Design review of the part built by this model. Coordinates are the model's own, in mm. Face numbers are marked on the shaded views. A direction names the side the tool comes from. Coordinates: 2 decimals unless noted, no trailing zeros. Write each loop counter-clockwise with the first axis right and the second up, starting at its lowest first coordinate (ties: lowest second). Pieces come first, ordered by that corner, then holes.
Q1. The part is to be moulded in two halves that separate along Z. For the marked faces 3, 4 and 5, say which applies: +Z half, -Z half, draft (parallel to the pull), parting line (faces both ways), or undercut.
Q2. Add section D-D, the plane y = 1.25. Give the boundary of the cut face in (x, z), plus the area to 3 significant figures.
Q3. Add section B-B, the plane y = 14.25. Give the boundary of the cut face in (x, z), plus the area to 3 significant figures.
Q4. Add section A-A, the plane x = 0. Give the boundary of the cut face in (y, z) (3 decimals), plus the area to 3 significant figures.
Q5. Clearance check with flat-ended pins moving along their axes: pin 1 Ø8 at (y, z) = (6, -4.5) entering from -X; pin 2 Ø7.5 at (y, z) = (16.5, 2.5) entering from +X; pin 3 Ø2 at (x, y) = (1.5, 12) entering from +Z. State where each tip first meets the part, or that it passes through.
Q6. To check wall thickness, follow probe 1 along Y at (x, z) = (-0.25, 0); probe 2 along Y at (x, z) = (2, -1.5); probe 3 along X at (y, z) = (3.75, -9). State the ranges of each line that lie inside material, in increasing order.
Q7. Machinability: for the marked faces 1 and 2, which of the approach directions +Z, -Z, +X, -X, +Y, -Y give a long, thin tool a straight path to every point of the face, cutting with its end or side? Answer none if there is none.
Q8. Add section C-C, the plane z = 0. Give the boundary of the cut face in (x, y) (3 decimals), plus the area to 3 significant figures.
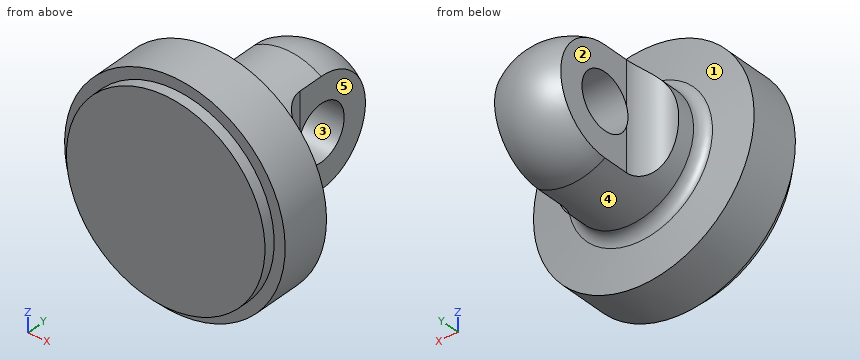
from build123d import *

# Parameters (mm, degrees)
CUT_EXTRUDE1_DEPTH      = 30.071628781
CUT_EXTRUDE1_DEPTH_BACK = 30.071628781
CUT_EXTRUDE2_DEPTH      = 31.926520981
CUT_EXTRUDE2_DEPTH_BACK = 31.926520981
SKETCH4_R               = 3.175


with BuildPart() as part:
    # Sketch1 → Revolve1 (revolve)
    with BuildSketch(Plane.XY, mode=Mode.PRIVATE) as revolve1_sk:
        with BuildLine():
            Line((-12.7, 0), (-12.7, 5.715))
            Line((-12.7, 5.715), (-8.325216792, 6.220171271))
            ThreePointArc((-8.325216792, 6.220171271), (-7.522765602, 6.636837464), (-7.2009, 7.481787854))
            Line((-7.2009, 7.481787854), (-7.2009, 15.6591))
            ThreePointArc((-7.2009, 15.6591), (-5.091805221, 20.750905221), (0, 22.86))
            Line((0, 22.86), (0, 6.35))
            Line((0, 6.35), (0, 0))
            Line((0, 0), (0, -1.27))
            Line((0, -1.27), (-11.43, -1.27))
            Line((-11.43, -1.27), (-11.43, 0))
            Line((-11.43, 0), (-12.7, 0))
        make_face()
    revolve(revolve1_sk.sketch.rotate(Axis((0, 6.35, 0), (0, -1, 0)), 270), axis=Axis((0, 6.35, 0), (0, -1, 0)))

    # Sketch3 → Cut-Extrude1 (cut, two sides: drawn at the far end of the back side and taken through both)
    with BuildSketch(Plane.XY.offset(-CUT_EXTRUDE1_DEPTH_BACK)):
        with BuildLine():
            Line((-3.81, 22.86), (-3.81, 12.7))
            ThreePointArc((-3.81, 12.7), (-6.985, 9.525), (-10.16, 12.7))
            Line((-10.16, 12.7), (-10.16, 22.86))
            Line((-10.16, 22.86), (-3.81, 22.86))
        make_face()
        with BuildLine():
            Line((10.16, 22.86), (10.16, 12.7))
            ThreePointArc((10.16, 12.7), (6.985, 9.525), (3.81, 12.7))
            Line((3.81, 12.7), (3.81, 22.86))
            Line((3.81, 22.86), (10.16, 22.86))
        make_face()
    extrude(amount=CUT_EXTRUDE1_DEPTH + CUT_EXTRUDE1_DEPTH_BACK, mode=Mode.SUBTRACT)

    # Sketch4 → Cut-Extrude2 (cut, two sides: drawn at the far end of the back side and taken through both)
    with BuildSketch(Plane.ZY.offset(3.81).offset(-CUT_EXTRUDE2_DEPTH_BACK)):
        with Locations(Location((0, 15.6591, 0), (0, 0, 248.748756024))):
            Circle(SKETCH4_R)
    extrude(amount=CUT_EXTRUDE2_DEPTH + CUT_EXTRUDE2_DEPTH_BACK, mode=Mode.SUBTRACT)


solid = part.part
Here are the results:
1. face 3: undercut
1. face 4: parting line
1. face 5: draft
2. outline: circle Ø25.4 at (0, 0)
2. area: 507 mm2
3. outline: (-3.81, -6.11) arc R7.2 ccw to (3.81, -6.11) - (3.81, -2.85) - (-3.81, -2.85) - close; (-3.81, 2.85) - (3.81, 2.85) - (3.81, 6.11) arc R7.2 ccw to (-3.81, 6.11) - close
3. area: 61.0 mm2
4. outline: (-1.27, -11.43) - (0, -11.43) - (0, -12.7) - (5.715, -12.7) - (6.22, -8.325) arc R1.27 cw to (7.482, -7.201) - (15.659, -7.201) arc R7.201 ccw to (15.659, 7.201) - (7.482, 7.201) arc R1.27 cw to (6.22, 8.325) - (5.715, 12.7) - (0, 12.7) - (0, 11.43) - (-1.27, 11.43) - close; hole circle Ø6.35 at (15.659, 0)
4. area: 371 mm2
5. pin 1: stops at x = -12.69
5. pin 2: stops at x = 3.81
5. pin 3: stops at z = 7.18
6. probe 1: y = -1.27 to 12.48, 18.83 to 22.86
6. probe 2: y = -1.27 to 12.86, 18.46 to 22.41
6. probe 3: x = -8.96 to 8.96
7. face 1: +Y
7. face 2: +Z, -Z, -X, +Y
8. outline: (-12.7, 0) - (-11.43, 0) - (-11.43, -1.27) - (11.43, -1.27) - (11.43, 0) - (12.7, 0) - (12.7, 5.715) - (8.325, 6.22) arc R1.27 cw to (7.201, 7.482) - (7.201, 9.532) arc R3.175 cw to (3.817, 12.484) - (-3.817, 12.484) arc R3.175 cw to (-7.201, 9.532) - (-7.201, 7.482) arc R1.27 cw to (-8.325, 6.22) - (-12.7, 5.715) - close; (-3.81, 18.834) - (3.81, 18.834) - (3.81, 21.769) arc R7.201 ccw to (-3.81, 21.769) - close
8. area: 288 mm2
